Can you work these out from the model? Positions are in its coordinate system, mm. A direction names the side the tool comes from. Round coordinates to 2 decimals unless told otherwise and drop trailing zeros. Loops run counter-clockwise (first coordinate to the right, second up) from the corner with the lowest first, then second, coordinate; pieces in that order, holes last. Notation, with made-up numbers: (84.5, 12.5) - (98.5, 12.5) arc R18 cw to (98.5, 33.5) - close; hole circle Ø8 at (13, 6.25). An arc over 180 degrees is marked (long way). Answer as CSV lines item,"result".
```python
from build123d import *

# Parameters (mm, degrees)
SKETCH1_R           = 15
BOSS_EXTRUDE1_DEPTH = 15
SKETCH4_W           = 28.284271248
SKETCH4_H           = 10
BOSS_EXTRUDE3_DEPTH = 17
FILLET3_R           = 5


with BuildPart() as part:
    # Sketch1 → Boss-Extrude1 (new body)
    with BuildSketch(Plane(origin=(0, 0, 0), x_dir=(1, 0, 0), z_dir=(0, 1, 0))):
        with Locations(Location((0, 0, 0), (0, 0, 270))):
            Circle(SKETCH1_R)
    extrude(amount=-BOSS_EXTRUDE1_DEPTH)

    # Sketch4 → Boss-Extrude3 (add)
    with BuildSketch(Plane(origin=(0, 0, 0), x_dir=(1, 0, 0), z_dir=(0, 1, 0))):
        Rectangle(SKETCH4_W, SKETCH4_H)
    extrude(amount=BOSS_EXTRUDE3_DEPTH)

    # Fillet3
    fillet3_edges = [part.edges().sort_by_distance(p)[0] for p in [
        (-14.142135624, 17, 0),
        (14.142135624, 17, 0),
    ]]
    fillet(fillet3_edges, radius=FILLET3_R)


solid = part.part
```
Q1. Imagine slicing it at B-B (x = 0). Write out the boundary of the cut face in (y, z).
Checks:
outline,"(-15, -15) - (0, -15) - (0, -5) - (17, -5) - (17, 5) - (0, 5) - (0, 15) - (-15, 15) - close"
Q2. I'm going to push flat-ended pins straight in: pin 1 Ø6 at (y, z) = (9.5, -8.5) entering from -X; pin 2 Ø10 at (y, z) = (11, -2) entering from +X; pin 3 Ø3 at (y, z) = (7.5, -2) entering from -X; pin 4 Ø5 at (x, y) = (-4.5, -4.5) entering from -Z. Where does each tip first touch, or does it pass through?
Checks:
pin 1,"through"
pin 2,"x = 14.14"
pin 3,"x = -14.14"
pin 4,"z = -14.87"
Q3. Imagine slicing it at A-A (z = 0). Write out the boundary of the cut face in (x, y), then the cut area to 3 significant figures.
Checks:
outline,"(-15, -15) - (15, -15) - (15, 0) - (14.14, 0) - (14.14, 12) arc R5 ccw to (9.14, 17) - (-9.14, 17) arc R5 ccw to (-14.14, 12) - (-14.14, 0) - (-15, 0) - close"
area,"920 mm²"
Q4. If I drill on line 1 along Y through (x, z) = (-10, -7); line 2 along X through (y, z) = (7, -4.5); line 3 along Z through (x, y) = (7.25, 7), over which ranges is the centre line in solid material (lowest first)? Write a range as [from, to].
Checks:
line 1,"[-15, 0]"
line 2,"[-14.14, 14.14]"
line 3,"[-5, 5]"
Q5. On a 3-axis mill with a long thin cutter (end or side, diameter ignored), from which of +Z, -Z, +X, -X, +Y, -Y can I reach the whole of each face in a straight line? I mean faces 1 (the flat face through (14.142, 6, 0)), 2 (the flat face through (0, 8, -5)), 3 (the flat face through (0, 0, 9)), 4 (the flat face through (-14.5, 0, -0.1)). Say none if no direction works.
Checks:
face 1,"+Z, -Z, +X, +Y"
face 2,"-Z, +X, -X, +Y"
face 3,"+Z, +X, -X, +Y"
face 4,"+Z, -Z, -X, +Y"
Q6. Imagine slicing it at C-C (y = -4.5). Write out the boundary of the cut face in (x, z), then the cut area to 3 significant figures.
Checks:
outline,"circle Ø30 at (0, 0)"
area,"707 mm²"
Q7. Imagine slicing it at D-D (z = -3). Write out the boundary of the cut face in (x, y), then the cut area to 3 significant figures.
Checks:
outline,"(-14.7, -15) - (14.7, -15) - (14.7, 0) - (14.14, 0) - (14.14, 12) arc R5 ccw to (9.14, 17) - (-9.14, 17) arc R5 ccw to (-14.14, 12) - (-14.14, 0) - (-14.7, 0) - close"
area,"911 mm²"
